Work out the finished part from the listing and answer in its coordinate system (mm). A direction names the side the tool comes from. Coordinates: 2 decimals unless noted, no trailing zeros. Order: outer loops, then holes, each group sorted by start corner. A loop starts at its lowest first (then second) coordinate and runs counter-clockwise, first axis right, second up.
```python
from build123d import *

# Parameters (mm, degrees)
F0_R     = 22.75
F1_DEPTH = 2
F2_R     = 4.4458772924
F3_DEPTH = 6
F4_R     = 4.4949655375
F5_DEPTH = 3
F6_R     = 1.0635
F7_DEPTH = 6
F8_R     = 1.0635
F9_DEPTH = 6


# Not quite as in the source:
# - a fillet or chamfer that OpenCascade refuses, or shapes differently, is made with other operations: its cross-section is extruded or revolved along the edge and cut away or added


with BuildPart() as f1:
    # F0 (on Front) → F1 (new body)
    with BuildSketch(Plane.XZ):
        Circle(F0_R)
    extrude(amount=F1_DEPTH)

    # F2 (on Front) → F3 (join)
    with BuildSketch(Plane.XZ):
        Circle(F2_R)
    extrude(amount=F3_DEPTH)

    # F4 (on Front) → F5 (join)
    with BuildSketch(Plane.XZ):
        Circle(F4_R)
    extrude(amount=-F5_DEPTH)

    # F6 (on Front) → F7 (cut)
    with BuildSketch(Plane.XZ):
        Circle(F6_R)
    extrude(amount=F7_DEPTH, mode=Mode.SUBTRACT)

    # F8 (on Front) → F9 (cut)
    with BuildSketch(Plane.XZ):
        Circle(F8_R)
    extrude(amount=-F9_DEPTH, mode=Mode.SUBTRACT)

    # F10: chamfer of 5 on 1 edges, made by hand

    # F10_s1 → F10_t2 (revolve, cut)
    with BuildSketch(Plane.XY):
        Polygon((22.75, 3), (17.75, -2), (22.75, -2), align=None)
    revolve(axis=Axis((0, -2, 0), (0, -1, 0)), mode=Mode.SUBTRACT)


solid = f1.part
```
1. Flat-ended cylindrical pins translate along their axes: pin 1 (5 mm diameter, centred on x = -7, z = 12, fed in from -Y); pin 2 (2 mm diameter, centred on x = 10, z = 4, fed in from +Y). Find the tip coordinate at first contact, or state that the pin passes through.
2. The part is cut by section D-D (y = -3.25). Determine the outline of the cut face in (x, z), plus the area to 3 significant figures.
3. Consider probe 1 along Z at (x, y) = (0, -4.6); probe 2 along Z at (x, y) = (0, 2.3); probe 3 along Y at (x, z) = (2.5, -13.5). Determine where each line is inside the solid, lowest interval first.
4. For faces 1 (the flat face through (1, -6, -1)), 2 (the cylindrical face through (-0.96, -3.97, -4.34)), 3 (the cylindrical face through (4.287, 1.479, 1.35)), determine the directions among +Z, -Z, +X, -X, +Y, -Y from which every point of the face is accessible in a straight line to the end or side of a thin tool.
5. The part is cut by section B-B (z = 0). Determine the outline of the cut face in (x, y), plus the area to 3 significant figures.
6. The part is cut by section C-C (y = -1.25). Determine the outline of the cut face in (x, z).
7. The part is cut by section A-A (x = 0). Determine the outline of the cut face in (y, z).
Worked out:
1. pin 1: stops at y = -2
1. pin 2: stops at y = 0
2. outline: circle Ø8.89 at (0, 0); hole circle Ø2.13 at (0, 0)
2. area: 58.5 mm2
3. probe 1: z = -4.45 to -1.06, 1.06 to 4.45
3. probe 2: z = -4.49 to -1.06, 1.06 to 4.49
3. probe 3: y = -2 to 0
4. face 1: +Z, -Z, +X, -X, -Y
4. face 2: -Y
4. face 3: +Y
5. outline: (-19.75, 0) - (-17.75, -2) - (-4.45, -2) - (-4.45, -6) - (-1.06, -6) - (-1.06, 3) - (-4.49, 3) - (-4.49, 0) - close; (1.06, -6) - (4.45, -6) - (4.45, -2) - (17.75, -2) - (19.75, 0) - (4.49, 0) - (4.49, 3) - (1.06, 3) - close
5. area: 118 mm2
6. outline: circle Ø37 at (0, 0); hole circle Ø2.13 at (0, 0)
7. outline: (-6, -4.45) - (-2, -4.45) - (-2, -17.75) - (0, -19.75) - (0, -4.49) - (3, -4.49) - (3, -1.06) - (-6, -1.06) - close; (-6, 1.06) - (3, 1.06) - (3, 4.49) - (0, 4.49) - (0, 19.75) - (-2, 17.75) - (-2, 4.45) - (-6, 4.45) - close
